Input: part model. Units: mm. Frame: model coordinates. A direction names the side the tool comes from. Give positions to 0.01 mm unless a question says otherwise; leave off trailing zeros. Loops run counter-clockwise (first coordinate to the right, second up) from the corner with the lowest first, then second, coordinate; pieces in that order, holes last. Notation, with made-up numbers: (21.25, -32) - (72.25, -32) arc R28 cw to (72.25, -8) - close; hole circle Ø11 at (-3, -16). An arc over 180 degrees is marked (long way). Answer as a JSON object with one key per item and string values.
Autodesk Inventor part; units mm, degrees
ref_plane "Work Plane1" through (0, 129.54, 0) normal (0, 1, 0) x (1, 0, 0)
ref_plane "YZ Plane" through (0, 0, 0) normal (1, 0, 0) x (0, 1, 0)
ref_plane "XZ Plane" through (0, 0, 0) normal (0, 1, 0) x (-1, 0, 0)
sketch "Sketch1" plane through (0, 0, 0) normal (0, 1, 0) x (-1, 0, 0)
  circle A0 centre (0, 0) radius 10.4775
  dimension "d0" = 20.955
extrude "Extrusion1" add sketch "Sketch1" along normal blind 95.25
sketch "Sketch2" plane through (0, 95.25, 0) normal (0, 1, 0) x (1, 0, 0)
  circle A0 centre (0, 0) radius 5.08
  dimension "d3" = 10.16
ref_plane "Work Plane1" through (0, 129.54, 0) normal (0, 1, 0) x (1, 0, 0)
sketch "Sketch3" plane through (0, 129.54, 0) normal (0, 1, 0) x (1, 0, 0)
  circle A0 centre (0, 0) radius 2.54
  dimension "d5" = 5.08
loft "Loft1" add profiles "Sketch2", "Sketch3"
sketch "Sketch4" plane through (0, 0, 0) normal (0, -1, 0) x (1, 0, 0)
  circle A0 centre (0, 0) radius 11.5507
  circle A1 centre (0, 11.5507) radius 7.1374
  circle A2 centre (0, -11.5507) radius 7.1374
  line L0 (7.1374, 11.5507) -> (11.5507, 0) construction
  line L1 (-7.1374, 11.5507) -> (-11.5507, 0) construction
  line L2 (-11.5507, 0) -> (-7.1374, -11.5507) construction
  line L3 (7.1374, -11.5507) -> (11.5507, 0) construction
  arc A3 (7.1374, 11.5507) -> (8.6078, 7.7021) centre (14.2137, 12.0492) ccw
  line L4 (11.5507, 0) -> (-11.5507, 0)
  line L5 (0, 11.5507) -> (0, -11.5507)
  arc A4 (-8.6078, 7.7021) -> (-7.1374, 11.5507) centre (-14.2137, 12.0492) ccw
  arc A5 (8.6078, -7.7021) -> (7.1374, -11.5507) centre (14.2137, -12.0492) ccw
  arc A6 (-7.1374, -11.5507) -> (-8.6078, -7.7021) centre (-14.2137, -12.0492) ccw
  circle A7 centre (0, 0) radius 11.5507
  dimension "d10" = 23.1013
  dimension "d11" = 14.2748
  dimension "d12" = 14.2748
extrude "Extrusion2" add sketch "Sketch4" against normal blind 2.032 contours L4 L5 A1 A0 | A0 A2 L5 L4 | L5 A2 A0 L4 | L4 A0 A1 L5 | A1 L5 A0 | A0 A1 | A2 A0 | A0 L5 A2 | A1 A0 L5 | L5 A0 A2
sketch "Sketch5" plane through (0, 0, 0) normal (0, -1, 0) x (1, 0, 0)
  circle A0 centre (0, 0) radius 5.08
  circle A1 centre (0, 0) radius 9.6202
  dimension "d15" = 19.2405
extrude "Extrusion3" cut sketch "Sketch5" against normal blind 93.5355 contours A0 | A1
properties part number "syringe"
Item 1: Access query for faces 1 (the face through (-0.188, 1.002, -18.686)), 2 (the face through (0, 93.536, 0)), 3 (the face through (1.36, 47.99, -10.39)). Directions: +Z, -Z, +X, -X, +Y, -Y. A direction counts if a zero-diameter tool reaches every point of the face in a straight line with its end or side. Return the directions, or none.
Geometry check:
{"face 1": "+Y, -Y", "face 2": "-Y", "face 3": "+Y"}
Item 2: Contact query for flat-ended pins moving along their axis: P1, Ø2, axis at y = 76.5, z = 9.5, coming from the +X side; P2, Ø10, axis at y = 64, z = -8, coming from the +X side; P3, Ø8, axis at x = -7.5, z = 14.5, coming from the +Y side. Output: stop coordinate, or through.
Geometry check:
{"P1": "stops at x = 6.13", "P2": "stops at x = 10.04", "P3": "stops at y = 2.03"}
Item 3: Cut plane B-B (x = 0). Return loops of the section in (y, z), then the cut area to 3 significant figures.
Geometry check:
{"outline": "(0, -18.69) - (2.03, -18.69) - (2.03, -10.48) - (95.25, -10.48) - (95.25, -5.08) - (129.54, -2.54) - (129.54, 2.54) - (95.25, 5.08) - (95.25, 10.48) - (2.03, 10.48) - (2.03, 18.69) - (0, 18.69) - (0, 9.62) - (93.54, 9.62) - (93.54, -9.62) - (0, -9.62) - close", "area": "491 mm2"}
Item 4: Cut plane A-A (y = 83). Return loops of the section in (x, z) (1 decimal).
Geometry check:
{"outline": "circle Ø21 at (0, 0); hole circle Ø19.2 at (0, 0)"}
Item 5: Cut plane C-C (z = -7.5). Return loops of the section in (x, y), then the cut area to 3 significant figures.
Geometry check:
{"outline": "(-8.78, 0) - (-6.02, 0) - (-6.02, 93.54) - (6.02, 93.54) - (6.02, 0) - (8.78, 0) - (8.78, 2.03) - (7.32, 2.03) - (7.32, 95.25) - (-7.32, 95.25) - (-7.32, 2.03) - (-8.78, 2.03) - close", "area": "273 mm2"}
Item 6: Cut plane D-D (y = 97). Return loops of the section in (x, z), then the cut area to 3 significant figures.
Geometry check:
{"outline": "circle Ø9.9 at (0, 0)", "area": "77.0 mm2"}
Item 7: Mould query, pull axis X, two halves, no side actions, for faces 4 (the face through (11.55, 1, -0.15)), 5 (the face through (-1.25, 46.11, 9.54)), 6 (the face through (2, 0, -10)). Classes: released by +X, released by -X, zero draft, split by the parting line, or undercut.
Geometry check:
{"face 4": "released by +X", "face 5": "undercut", "face 6": "zero draft"}
Item 8: Material intervals for line 1 (Z direction, x = 0, y = 47); line 2 (Y direction, x = 2, z = 8.5); line 3 (Y direction, x = -2.5, z = -16.5), sorted ascending. Write a range as [from, to].
Geometry check:
{"line 1": "z = [-10.48, -9.62], [9.62, 10.48]", "line 2": "y = [93.54, 95.25]", "line 3": "y = [0, 2.03]"}
